Can you work these out from the drawing? Everything is in mm from the part's minimum corner. Round coordinates to 2 decimals unless told otherwise and drop trailing zeros. Loops run counter-clockwise (first coordinate to the right, second up) from the corner with the lowest first, then second, coordinate; pieces in that order, holes last. Notation, with made-up numbers: (-20, -26.5) -> (-11, -26.5) arc R12 cw to (-11, -7.5) -> close; hole circle Ø10 at (44.25, 87.5). An arc over 180 degrees is marked (long way). One line per item, written item: value.
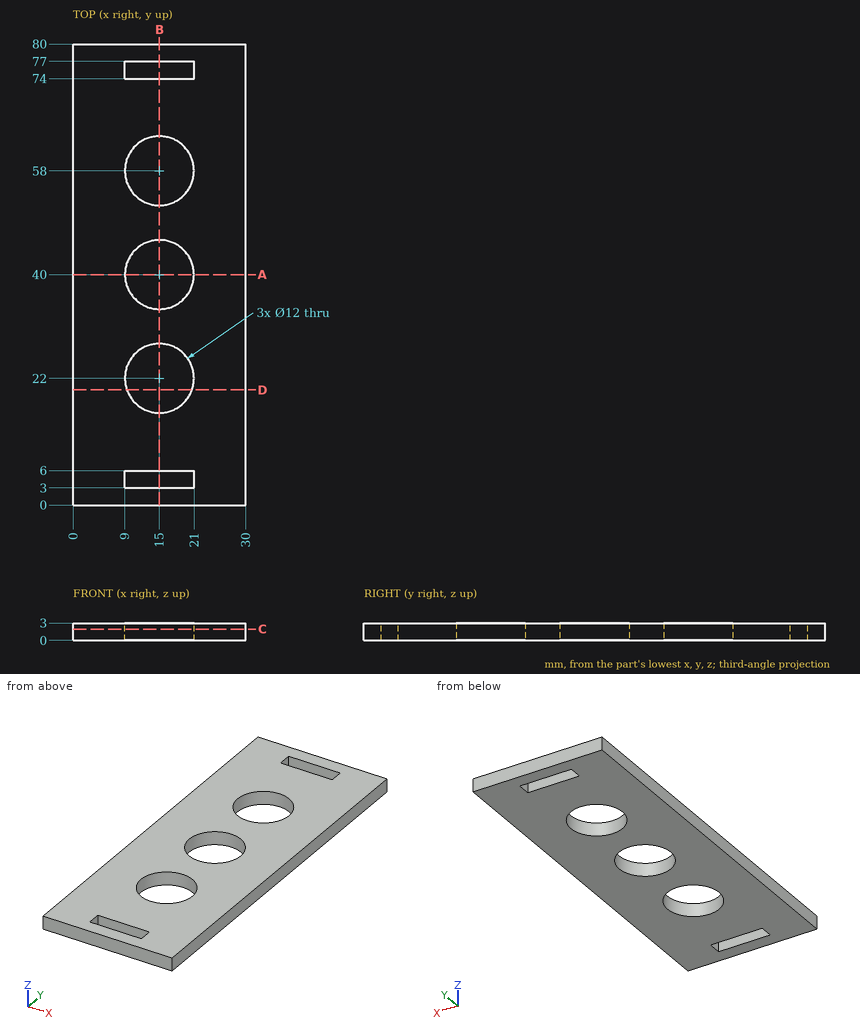
Item 1: If we section it at B-B on x = 15: List the corners of the cut face in (y, z) for me.
Output:
outline: (0, 0) -> (3, 0) -> (3, 3) -> (0, 3) -> close; (6, 0) -> (16, 0) -> (16, 3) -> (6, 3) -> close; (28, 0) -> (34, 0) -> (34, 3) -> (28, 3) -> close; (46, 0) -> (52, 0) -> (52, 3) -> (46, 3) -> close; (64, 0) -> (74, 0) -> (74, 3) -> (64, 3) -> close; (77, 0) -> (80, 0) -> (80, 3) -> (77, 3) -> close
Item 2: If we section it at D-D on y = 20: List the corners of the cut face in (x, z) for me.
Output:
outline: (0, 0) -> (9.34, 0) -> (9.34, 3) -> (0, 3) -> close; (20.66, 0) -> (30, 0) -> (30, 3) -> (20.66, 3) -> close
Item 3: I need wall thicknesses on line 1 (Y direction, x = 15, z = 0.9); line 2 (X direction, y = 22, z = 2.2); line 3 (Y direction, x = 20, z = 1.2). Which ranges of each line are inside material? Lowest first, please. Write a range as from..to.
Output:
line 1: y = 0..3, 6..16, 28..34, 46..52, 64..74, 77..80
line 2: x = 0..9, 21..30
line 3: y = 0..3, 6..18.68, 25.32..36.68, 43.32..54.68, 61.32..74, 77..80
Item 4: If we section it at C-C on z = 1.95: List the corners of the cut face in (x, y) for me, plus the area to 3 significant figures.
Output:
outline: (0, 0) -> (30, 0) -> (30, 80) -> (0, 80) -> close; hole (9, 3) -> (21, 3) -> (21, 6) -> (9, 6) -> close; hole circle Ø12 at (15, 22); hole circle Ø12 at (15, 40); hole circle Ø12 at (15, 58); hole (9, 74) -> (21, 74) -> (21, 77) -> (9, 77) -> close
area: 1,990 mm²
Item 5: If we section it at A-A on y = 40: List the corners of the cut face in (x, z) for me, plus the area to 3 significant figures.
Output:
outline: (0, 0) -> (9, 0) -> (9, 3) -> (0, 3) -> close; (21, 0) -> (30, 0) -> (30, 3) -> (21, 3) -> close
area: 54.0 mm²
